Read the model definition and answer for the solid it produces. Units are mm, in the model's axes. A direction names the side the tool comes from. Give positions to 0.01 mm unless a question says otherwise; leave off trailing zeros. Write each loop counter-clockwise with the first axis right and the second up, starting at its lowest first coordinate (ties: lowest second). Pieces come first, ordered by that corner, then holes. Notation, with made-up numbers: M -4,16.25 L 51,16.25 A24 ccw 51,49.25 Z; hole C 5,16 d10. An arc over 180 degrees is marked long. Write each question's results on one line, items separated by ' | '. Start each with the question number.
```python
from build123d import *

# Parameters (mm, degrees)
SKETCH1_R           = 9.5
BOSS_EXTRUDE1_DEPTH = 1.75
BOSS_EXTRUDE4_START = -1.75
BOSS_EXTRUDE4_DEPTH = 1.75
SKETCH2_R           = 1.6
CUT_EXTRUDE1_DEPTH  = 1.75
SKETCH3_W           = 4.4
SKETCH3_H           = 4.4
BOSS_EXTRUDE2_DEPTH = 1.05
SKETCH4_R           = 1.7
BOSS_EXTRUDE3_DEPTH = 1.7
FILLET1_R           = 1.7


with BuildPart() as part:
    # Sketch1 → Boss-Extrude1 (new body)
    with BuildSketch(Plane(origin=(0, 0, 0), x_dir=(1, 0, 0), z_dir=(0, 1, 0))):
        with Locations(Location((0, 0, 0), (0, 0, 270))):
            Circle(SKETCH1_R)
    extrude(amount=BOSS_EXTRUDE1_DEPTH)

    # Sketch5 → Boss-Extrude4 (add)
    with BuildSketch(Plane(origin=(0, 1.75, 0), x_dir=(1, 0, 0), z_dir=(0, 1, 0)).offset(BOSS_EXTRUDE4_START)):
        with BuildLine():
            Line((-1.949608457, 10.363663389), (-8.000391543, 6.870242146))
            Line((-8.000391543, 6.870242146), (-7.44257413, 5.904074045))
            ThreePointArc((-7.44257413, 5.904074045), (-4.75, 8.227241336), (-1.391791044, 9.397495288))
            Line((-1.391791044, 9.397495288), (-1.949608457, 10.363663389))
        make_face()
        with BuildLine():
            ThreePointArc((-8.834365173, -3.493421243), (-9.5, 0), (-8.834365173, 3.493421243))
            Line((-8.834365173, 3.493421243), (-9.95, 3.493421243))
            Line((-9.95, 3.493421243), (-9.95, -3.493421243))
            Line((-9.95, -3.493421243), (-8.834365173, -3.493421243))
        make_face()
        with BuildLine():
            Line((1.949608457, 10.363663389), (1.391791044, 9.397495288))
            ThreePointArc((1.391791044, 9.397495288), (4.75, 8.227241336), (7.44257413, 5.904074045))
            Line((7.44257413, 5.904074045), (8.000391543, 6.870242146))
            Line((8.000391543, 6.870242146), (1.949608457, 10.363663389))
        make_face()
        with BuildLine():
            ThreePointArc((-1.391791044, -9.397495288), (-4.75, -8.227241336), (-7.44257413, -5.904074045))
            Line((-7.44257413, -5.904074045), (-8.000391543, -6.870242146))
            Line((-8.000391543, -6.870242146), (-1.949608457, -10.363663389))
            Line((-1.949608457, -10.363663389), (-1.391791044, -9.397495288))
        make_face()
        with BuildLine():
            Line((9.95, 3.493421243), (8.834365173, 3.493421243))
            ThreePointArc((8.834365173, 3.493421243), (9.5, 0), (8.834365173, -3.493421243))
            Line((8.834365173, -3.493421243), (9.95, -3.493421243))
            Line((9.95, -3.493421243), (9.95, 3.493421243))
        make_face()
        with BuildLine():
            ThreePointArc((7.44257413, -5.904074045), (4.75, -8.227241336), (1.391791044, -9.397495288))
            Line((1.391791044, -9.397495288), (1.949608457, -10.363663389))
            Line((1.949608457, -10.363663389), (8.000391543, -6.870242146))
            Line((8.000391543, -6.870242146), (7.44257413, -5.904074045))
        make_face()
    extrude(amount=BOSS_EXTRUDE4_DEPTH)

    # Sketch2 → Cut-Extrude1 (cut)
    with BuildSketch(Plane(origin=(0, 1.75, 0), x_dir=(1, 0, 0), z_dir=(0, 1, 0))):
        with Locations((0, -9.5)):
            Circle(SKETCH2_R)
        with Locations((-8.213474399, -4.742078212)):
            Circle(SKETCH2_R)
        with Locations((-8.199730461, 4.749960166)):
            Circle(SKETCH2_R)
        with Locations((0.027487877, 9.484076755)):
            Circle(SKETCH2_R)
        with Locations((8.240962276, 4.726154966)):
            Circle(SKETCH2_R)
        with Locations((8.227218338, -4.765883411)):
            Circle(SKETCH2_R)
    extrude(amount=-CUT_EXTRUDE1_DEPTH, mode=Mode.SUBTRACT)

    # Sketch3 → Boss-Extrude2 (add)
    with BuildSketch(Plane(origin=(0, 1.75, 0), x_dir=(1, 0, 0), z_dir=(0, 1, 0))):
        Rectangle(SKETCH3_W, SKETCH3_H)
    extrude(amount=BOSS_EXTRUDE2_DEPTH)

    # Sketch4 → Boss-Extrude3 (add)
    with BuildSketch(Plane(origin=(0, 2.8, 0), x_dir=(1, 0, 0), z_dir=(0, 1, 0))):
        with Locations(Location((0, 0, 0), (0, 0, 270))):
            Circle(SKETCH4_R)
    extrude(amount=BOSS_EXTRUDE3_DEPTH)

    # Fillet1
    fillet1_edges = [part.edges().sort_by_distance(p)[0] for p in [
        (0, 4.5, -1.7),
    ]]
    fillet(fillet1_edges, radius=FILLET1_R - 0.0001)  # a hair under: the kernel refuses the full size


solid = part.part
```
Item 1: Given P1, Ø0.6, axis at x = -9.5, y = 0.5, coming from the +Z side; P2, Ø1.5, axis at y = 1, z = -4.5, coming from the +X side; P3, Ø1, axis at y = 3, z = 1.5, coming from the -X side, each flat-ended and moving along its own axis, determine where each tip first touches the part or whether it passes through.
Item 2: Straight lines are drawn through the part: line 1 (Z direction, x = 7, y = 1.25); line 2 (Y direction, x = -4.25, z = -6.5); line 3 (Z direction, x = 0, y = 0.4). For each, find the intervals that lie inside material, in ascending order.
Item 3: Section B-B, the plane z = 2.5 is taken. Determine the outline of the cut face in (x, y), then the cut area to 3 significant figures.
Item 4: For faces 4 (the flat face through (0, 2, 2.2)), 5 (the cylindrical face through (-6.824, 0.887, -3.933)), 6 (the flat face through (-2.2, 2, 0)), determine the directions among +Z, -Z, +X, -X, +Y, -Y from which every point of the face is accessible in a straight line to the end or side of a thin tool.
Item 5: Section C-C, the plane x = 5.25 is taken. Determine the outline of the cut face in (y, z).
Item 6: Section A-A, the plane y = 1.35 is taken. Determine the outline of the cut face in (x, z).
Item 7: Determine the mould class of faces 1 (the cylindrical face through (6.85, 0.89, 3.95)), 2 (the flat face through (9.95, 1, 0)), 3 (the flat face through (4.933, 0.863, 8.641)) for opening direction Z: +Z half, -Z half, draft (parallel to the pull), parting line (faces both ways), or undercut.
Worked out:
1) P1: stops at z = 3.49 | P2: stops at x = 6.97 | P3: stops at x = -2.2
2) line 1: z = -7.45 to -5.74, -3.72 to 3.74, 5.79 to 7.45 | line 2: y = 0 to 1.75 | line 3: z = -7.88 to 7.9
3) outline: M -9.95,0 L 9.95,0 L 9.95,1.75 L -9.95,1.75 Z | area: 34.8 mm²
4) face 4: +Z, +X, -X, +Y | face 5: +Y, -Y | face 6: +Z, -Z, -X, +Y
5) outline: M 0,-8.46 L 1.75,-8.46 L 1.75,8.46 L 0,8.46 Z
6) outline: M -9.95,-3.49 L -9.19,-3.49 A1.6 cw long -7.64,-6.25 L -8,-6.87 L -1.95,-10.36 L -1.56,-9.69 A1.6 cw long 1.6,-9.76 L 1.95,-10.36 L 8,-6.87 L 7.61,-6.2 A1.6 cw long 9.26,-3.49 L 9.95,-3.49 L 9.95,3.49 L 9.2,3.49 A1.6 cw long 7.65,6.26 L 8,6.87 L 1.95,10.36 L 1.58,9.73 A1.6 cw long -1.58,9.73 L -1.95,10.36 L -8,6.87 L -7.63,6.23 A1.6 cw long -9.21,3.49 L -9.95,3.49 Z
7) face 1: undercut | face 2: draft | face 3: +Z half
